```python
from build123d import *

# Parameters (mm, degrees)
F0_W     = 75.528022
F0_H     = 64.241523
F1_DEPTH = 1
F2_W     = 1
F2_H     = 50
F3_DEPTH = 25


with BuildPart() as f1:
    # F0 (on Front) → F1 (new body)
    with BuildSketch(Plane.XZ):
        with Locations((-5.417621, 16.441694)):
            Rectangle(F0_W, F0_H)
    extrude(amount=F1_DEPTH)

    # F2 (on face) → F3 (join, symmetric)
    with BuildSketch(Plane.XZ.offset(1)):
        with Locations((-7.686447, 14.69165)):
            Rectangle(F2_W, F2_H)
    extrude(amount=F3_DEPTH, both=True)


solid = f1.part
```
Verification items for the finished model (mm, model axes). A direction names the side the tool comes from. Give positions to 0.01 mm unless a question says otherwise; leave off trailing zeros. Order: outer loops, then holes, each group sorted by start corner. A loop starts at its lowest first (then second) coordinate and runs counter-clockwise, first axis right, second up. Notation, with made-up numbers: M -9.5,78 L 27.5,78 A16 cw 27.5,100 Z; hole C -12,75 d7. An arc over 180 degrees is marked long. Return JSON: item names as keys, results as strings. Group by question number.
1) Scan lines: line 1 (X direction, y = -19, z = 36.5); line 2 (Y direction, x = 8, z = 28). Record each from-to range of solid material in increasing order.
2) Section check B-B on y = 21. Record the cut outline in (x, z).
3) Section check C-C on x = -33. Record the cut outline in (y, z), and give its area (3 significant figures).
4) Section check A-A on z = 21. Record the cut outline in (x, y).
5) Go/stop test with flat-tipped pins: pin 1 Ø1.1 at (x, y) = (-8, -14) entering from +Z; pin 2 Ø6 at (x, z) = (16.5, 12) entering from -Y; pin 3 Ø7 at (y, z) = (8, 16.5) entering from -X; pin 4 Ø12 at (x, y) = (-16.5, 11.5) entering from -Z. Record where each tip stops, or that it passes through.
6) Access from +Z, -Z, +X, -X, +Y, -Y to the whole of each face (thin tool, end or side, straight path). Record for faces 1 (the face through (-8.186, -14, 14)), 2 (the face through (-7.186, 12, 14)), 3 (the face through (-7.186, -14, 14)).
Answer block:
{
 "1": {"line 1": "x = -8.19 to -7.19", "line 2": "y = -1 to 0"},
 "2": {"outline": "M -8.19,-10.31 L -7.19,-10.31 L -7.19,39.69 L -8.19,39.69 Z"},
 "3": {"outline": "M -1,-15.68 L 0,-15.68 L 0,48.56 L -1,48.56 Z", "area": "64.2 mm^2"},
 "4": {"outline": "M -43.18,-1 L -8.19,-1 L -8.19,-26 L -7.19,-26 L -7.19,-1 L 32.35,-1 L 32.35,0 L -7.19,0 L -7.19,24 L -8.19,24 L -8.19,0 L -43.18,0 Z"},
 "5": {"pin 1": "stops at z = 39.69", "pin 2": "stops at y = -1", "pin 3": "stops at x = -8.19", "pin 4": "passes through"},
 "6": {"face 1": "+Z, -Z, -X, -Y", "face 2": "+Z, -Z, +X, +Y", "face 3": "+Z, -Z, +X, -Y"}
}
